```python
from build123d import *

# Parameters (mm, degrees)
CYLINDER259_R               = 2
CYLINDER259_DEPTH           = 10
CYLINDER259_PLACEMENT_ANGLE = 45
CYLINDER258_R               = 3
CYLINDER258_DEPTH           = 37
CYLINDER254_R               = 0.5
CYLINDER254_DEPTH           = 10
CYLINDER253_R               = 2
CYLINDER253_DEPTH           = 4
CYLINDER257_R               = 3
CYLINDER257_DEPTH           = 10
BOX138_W                    = 10
BOX138_H                    = 10
BOX138_DEPTH                = 10
BOX136_W                    = 2
BOX136_H                    = 10
BOX136_DEPTH                = 10
BOX137_W                    = 10
BOX137_H                    = 10
BOX137_DEPTH                = 10
CYLINDER256_R               = 5
CYLINDER256_DEPTH           = 10
CYLINDER255_R               = 5
CYLINDER255_DEPTH           = 10
BOX133_W                    = 10
BOX133_H                    = 10
BOX133_DEPTH                = 20
BOX133_PLACEMENT_ANGLE      = 30
BOX134_W                    = 12
BOX134_H                    = 10
BOX134_DEPTH                = 17
BOX134_PLACEMENT_ANGLE      = 30
BOX135_W                    = 12.5
BOX135_H                    = 10
BOX135_DEPTH                = 43


with BuildPart() as cylinder259:
    # Cylinder259 → Cylinder259 (new body)
    with BuildSketch(Plane.XY):
        Circle(CYLINDER259_R)
    extrude(amount=CYLINDER259_DEPTH)


with BuildPart() as cylinder259_1:
    # Cylinder259 placement: moved
    add(cylinder259.part.moved(Location((-62.041631, 0, -84.020815))).rotate(Axis((-62.041631, 0, -84.020815), (0, 1, 0)), CYLINDER259_PLACEMENT_ANGLE))


with BuildPart() as cylinder258:
    # Cylinder258 → Cylinder258 (new body)
    with BuildSketch(Plane(origin=(-52, 0, -84.5), x_dir=(1, 0, 0), z_dir=(0, 0, 1))):
        Circle(CYLINDER258_R)
    extrude(amount=CYLINDER258_DEPTH)


with BuildPart() as cylinder254:
    # Cylinder254 → Cylinder254 (new body)
    with BuildSketch(Plane(origin=(-5, 0, -7), x_dir=(0, 0, -1), z_dir=(1, 0, 0))):
        Circle(CYLINDER254_R)
    extrude(amount=CYLINDER254_DEPTH)


with BuildPart() as cylinder253:
    # Cylinder253 → Cylinder253 (new body)
    with BuildSketch(Plane(origin=(-2, -50, 1), x_dir=(0, 0, -1), z_dir=(1, 0, 0))):
        Circle(CYLINDER253_R)
    extrude(amount=CYLINDER253_DEPTH)


with BuildPart() as cylinder257:
    # Cylinder257 → Cylinder257 (new body)
    with BuildSketch(Plane(origin=(0, -50, -12), x_dir=(1, 0, 0), z_dir=(0, 0, 1))):
        Circle(CYLINDER257_R)
    extrude(amount=CYLINDER257_DEPTH)


with BuildPart() as cube138:
    # Box138 → Box138 (new body)
    with BuildSketch(Plane(origin=(-12, -55, -2), x_dir=(1, 0, 0), z_dir=(0, 0, 1))):
        with Locations((5, 5)):
            Rectangle(BOX138_W, BOX138_H)
    extrude(amount=BOX138_DEPTH)


with BuildPart() as cube136:
    # Box136 → Box136 (new body)
    with BuildSketch(Plane(origin=(-1, -55, -2), x_dir=(1, 0, 0), z_dir=(0, 0, 1))):
        with Locations((1, 5)):
            Rectangle(BOX136_W, BOX136_H)
    extrude(amount=BOX136_DEPTH)


with BuildPart() as cube137:
    # Box137 → Box137 (new body)
    with BuildSketch(Plane(origin=(2, -55, -2), x_dir=(1, 0, 0), z_dir=(0, 0, 1))):
        with Locations((5, 5)):
            Rectangle(BOX137_W, BOX137_H)
    extrude(amount=BOX137_DEPTH)


with BuildPart() as cylinder256:
    # Cylinder256 → Cylinder256 (new body)
    with BuildSketch(Plane(origin=(0, -50, -10), x_dir=(1, 0, 0), z_dir=(0, 0, 1))):
        Circle(CYLINDER256_R)
    extrude(amount=CYLINDER256_DEPTH)


with BuildPart() as sphere049:
    # Sphere049 → Sphere049 (revolve)
    with BuildSketch(Plane.XZ.offset(50)):
        with BuildLine():
            ThreePointArc((5, 0), (3.535534, 3.535534), (0, 5))
            Line((0, 5), (0, 0))
            Line((0, 0), (5, 0))
        make_face()
    revolve(axis=Axis((0, -50, 0), (0, 0, 1)))


with BuildPart() as cut204006062:
    # Cylinder255 → Cylinder255 (new body)
    with BuildSketch(Plane(origin=(0, -50, -7), x_dir=(1, 0, 0), z_dir=(0, 0, 1))):
        Circle(CYLINDER255_R)
    extrude(amount=CYLINDER255_DEPTH)

    # Common042: intersect Sphere049
    add(sphere049.part, mode=Mode.INTERSECT)

    # Fusion005077020026: union Cylinder256
    add(cylinder256.part)

    # Cut204006061: cut Cube137
    add(cube137.part, mode=Mode.SUBTRACT)

    # Cut204006063: cut Cube136
    add(cube136.part, mode=Mode.SUBTRACT)

    # Cut204006064: cut Cube138
    add(cube138.part, mode=Mode.SUBTRACT)

    # Cut204006060: cut Cylinder257
    add(cylinder257.part, mode=Mode.SUBTRACT)

    # Fusion005077020025: union Cylinder253
    add(cylinder253.part)


with BuildPart() as cut204006062_1:
    # Fusion005077020027 placement: moved
    add(cut204006062.part.moved(Location((0, 50, -8.5))))

    # Cut204006062: cut Cylinder254
    add(cylinder254.part, mode=Mode.SUBTRACT)


with BuildPart() as cut204006062_2:
    # Cut204006062 placement: moved
    add(cut204006062_1.part.moved(Location((-52, 0, -37))))


with BuildPart() as cube133:
    # Box133 → Box133 (new body)
    with BuildSketch(Plane.XY):
        with Locations((5, 5)):
            Rectangle(BOX133_W, BOX133_H)
    extrude(amount=BOX133_DEPTH)


with BuildPart() as cube133_1:
    # Box133 placement: moved
    add(cube133.part.moved(Location((-168.49167, -5, -108.102886))).rotate(Axis((-168.49167, -5, -108.102886), (0, -1, 0)), BOX133_PLACEMENT_ANGLE))


with BuildPart() as cube134:
    # Box134 → Box134 (new body)
    with BuildSketch(Plane.XY):
        with Locations((6, 5)):
            Rectangle(BOX134_W, BOX134_H)
    extrude(amount=BOX134_DEPTH)


with BuildPart() as cube134_1:
    # Box134 placement: moved
    add(cube134.part.moved(Location((-167.14, -5, -90.45))).rotate(Axis((-167.14, -5, -90.45), (0, -1, 0)), BOX134_PLACEMENT_ANGLE))


with BuildPart() as cut204006066:
    # Box135 → Box135 (new body)
    with BuildSketch(Plane(origin=(-168, -5, -90.5), x_dir=(1, 0, 0), z_dir=(0, 0, 1))):
        with Locations((6.25, 5)):
            Rectangle(BOX135_W, BOX135_H)
    extrude(amount=BOX135_DEPTH)

    # Fusion005077020024: union Cube134
    add(cube134_1.part)

    # Cut204006058: cut Cube133
    add(cube133_1.part, mode=Mode.SUBTRACT)


with BuildPart() as cut204006066_1:
    # Cut204006059 placement: moved
    add(cut204006066.part.moved(Location((110, 0, 0))))

    # Fusion005077020028: union Cut204006062
    add(cut204006062_2.part)

    # Cut204006065: cut Cylinder258
    add(cylinder258.part, mode=Mode.SUBTRACT)

    # Cut204006066: cut Cylinder259
    add(cylinder259_1.part, mode=Mode.SUBTRACT)


with BuildPart() as cut204006066_2:
    # Cut204006066 placement: moved
    add(cut204006066_1.part.moved(Location((153.5, 0, 0))))


solid = cut204006066_2.part
```
Design review of the part built by this model. Coordinates are the model's own, in mm. A direction names the side the tool comes from. Coordinates: 2 decimals unless noted, no trailing zeros. Write each loop counter-clockwise with the first axis right and the second up, starting at its lowest first coordinate (ties: lowest second). Pieces come first, ordered by that corner, then holes. Notation, with made-up numbers: M 29,35 L 58,35 A23 ccw 58,59 Z; hole C -21.75,-21.5 d4. An arc over 180 degrees is marked long. Answer as a JSON object with one key per item and string values.
Item 1: Add section D-D, the plane z = -87.5. Give the boundary of the cut face in (x, y).
Outcome:
{"outline": "M 94.66,-5 L 108,-5 L 108,5 L 94.66,5 Z"}
Item 2: Machinability: for faces 4 (the flat face through (100, 0, -47.5)), 5 (the cylindrical face through (99.985, -4.765, -46.514)), 6 (the cylindrical face through (103.015, 4.765, -46.514)), 7 (the cylindrical face through (100, 4.77, -46.51)), 8 (the flat face through (99.5, 0, -45)), which of the approach directions +Z, -Z, +X, -X, +Y, -Y give a long, thin tool a straight path to every point of the face, cutting with its end or side? Answer none if there is none.
Outcome:
{"face 4": "none", "face 5": "+Z, -X, -Y", "face 6": "+Z, +X, +Y", "face 7": "+Z, -X, +Y", "face 8": "+Z, -X, +Y, -Y"}
Item 3: Add section A-A, the plane x = 101.5. Give the boundary of the cut face in (y, z), and give its area (3 significant figures).
Outcome:
{"outline": "M -5,-90.5 L 5,-90.5 L 5,-47.5 L 3,-47.5 L 3,-84.5 L -3,-84.5 L -3,-47.5 L -5,-47.5 Z; C 0,-44.5 d4; hole C 0,-44 d1", "area": "220 mm²"}
Item 4: Add section C-C, the plane x = 106. Give the boundary of the cut face in (y, z).
Outcome:
{"outline": "M -5,-90.5 L 5,-90.5 L 5,-47.5 L -5,-47.5 Z"}
Item 5: Insertion check: pin 1 Ø5 at (y, z) = (3, -67) entering from -X; pin 2 Ø2.5 at (y, z) = (-2.5, -45) entering from -X; pin 3 Ø4 at (y, z) = (0.5, -44.5) entering from +X; pin 4 Ø6 at (x, z) = (91.5, -57.5) entering from -Y. Each pin has a flat end and moves straight along its axis. Give the tip position at first contact, or say it passes through.
Outcome:
{"pin 1": "x = 95.5", "pin 2": "x = 99.5", "pin 3": "x = 103.5", "pin 4": "through"}
Item 6: Add section B-B, the plane z = -70. Give the boundary of the cut face in (x, y).
Outcome:
{"outline": "M 95.5,-5 L 108,-5 L 108,5 L 95.5,5 Z; hole C 101.5,0 d6"}
Item 7: Draft analysis for pull direction Y (two halves, no side actions). For faces 1 (the flat face through (98.1, 0.03, -76.52)), 2 (the flat face through (100, 5, -69)), 3 (the flat face through (100, 0, -42.5)), state which applies: pulls with the +Y half, pulls with the -Y half, needs draft (parallel to the pull), parting line crosses it, or undercut.
Outcome:
{"face 1": "undercut", "face 2": "pulls with the +Y half", "face 3": "needs draft"}
Item 8: Wall thickness on probe 1 along X at (y, z) = (0, -70.5); probe 2 along Y at (x, z) = (101.5, -59); probe 3 along X at (y, z) = (0, -75): over which ranges is each line inside the solid? List them lowest first.
Outcome:
{"probe 1": "95.5 to 98.5, 104.5 to 108", "probe 2": "-5 to -3, 3 to 5", "probe 3": "89.12 to 98.5, 104.5 to 108"}
